```python
from build123d import *

# Parameters (mm, degrees)
SKETCH1_W                                       = 317.5
SKETCH1_H                                       = 50.8
BOSS_EXTRUDE1_DEPTH                             = 6.35
CBORE_FOR_10_SOCKET_HEAD_CAP_SCREW1_D           = 5.1054
CBORE_FOR_10_SOCKET_HEAD_CAP_SCREW1_CBORE_D     = 9.525
CBORE_FOR_10_SOCKET_HEAD_CAP_SCREW1_CBORE_DEPTH = 4.826
CBORE_FOR_10_SOCKET_HEAD_CAP_SCREW2_D           = 5.1054
CBORE_FOR_10_SOCKET_HEAD_CAP_SCREW2_CBORE_D     = 9.525
CBORE_FOR_10_SOCKET_HEAD_CAP_SCREW2_CBORE_DEPTH = 4.826
F_1_4_20_TAPPED_HOLE1_OUTLINE_R                 = 2.5527
F_1_4_20_TAPPED_HOLE1_DEPTH                     = 6.35


# Read off the part's stored shape, not the designer's step: 1/4-20 Tapped Hole1
with BuildPart() as part:
    # Sketch1 → Boss-Extrude1 (new body)
    with BuildSketch(Plane(origin=(0, 0, 0), x_dir=(1, 0, 0), z_dir=(0, 1, 0))):
        Rectangle(SKETCH1_W, SKETCH1_H)
    extrude(amount=BOSS_EXTRUDE1_DEPTH)

    # CBORE for #10 Socket Head Cap Screw1 (through all)
    with Locations(Plane(origin=(0, 6.35, 0), x_dir=(1, 0, 0), z_dir=(0, 1, 0))):
        with Locations((-125.73, -5.08), (19.05, 12.7), (69.85, 12.7), (19.05, -12.7), (69.85, -12.7), (-125.73, 15.24), (-125.73, 5.08), (-125.73, -15.24)):
            CounterBoreHole(CBORE_FOR_10_SOCKET_HEAD_CAP_SCREW1_D / 2, CBORE_FOR_10_SOCKET_HEAD_CAP_SCREW1_CBORE_D / 2, CBORE_FOR_10_SOCKET_HEAD_CAP_SCREW1_CBORE_DEPTH)

    # CBORE for #10 Socket Head Cap Screw2 (through all)
    with Locations(Plane.XZ):
        with Locations((-146.05, 12.7), (-146.05, 0), (-146.05, -12.7), (146.05, 12.7), (146.05, 0), (146.05, -12.7)):
            CounterBoreHole(CBORE_FOR_10_SOCKET_HEAD_CAP_SCREW2_D / 2, CBORE_FOR_10_SOCKET_HEAD_CAP_SCREW2_CBORE_D / 2, CBORE_FOR_10_SOCKET_HEAD_CAP_SCREW2_CBORE_DEPTH)

    # 1/4-20 Tapped Hole1 outline → 1/4-20 Tapped Hole1 (cut)
    with BuildSketch(Plane(origin=(0, 0, 0), x_dir=(1, 0, 0), z_dir=(0, 1, 0))):
        with Locations((-57.15, 20.32)):
            Circle(F_1_4_20_TAPPED_HOLE1_OUTLINE_R)
    extrude(amount=F_1_4_20_TAPPED_HOLE1_DEPTH, mode=Mode.SUBTRACT)


solid = part.part
```
CAD build for the part. Positions are in the model's coordinates, mm. A direction names the side the tool comes from. Round coordinates to 2 decimals unless told otherwise and drop trailing zeros. Write item = value, one per line. Start each with the question number.
Q1. Mould opens along X. For faces 1 (the flat face through (-2, 6.35, 0)), 2 (the cylindrical face through (-148.485, 5.599, 13.467)), 3 (the cylindrical face through (-123.18, 0.75, 4.97)) say: pulls with the +X half, pulls with the -X half, needs draft (parallel to the pull), parting line crosses it, or undercut.
Q2. Drop flat-ended pins along their axis: pin 1 (8.5 mm diameter, centred on x = 19.05, z = 12.7, fed in from +Y); pin 2 (8 mm diameter, centred on x = 146.05, z = -12.7, fed in from -Y). Give the stop position or say it passes through.
Q3. Probe L1, parallel to Z at x = 146.05, y = 1.45; L2, parallel to Z at x = 69.85, y = 4.7; L3, parallel to Z at x = -125.73, y = 2.8. List the from-to ranges inside material, lowest first. Write a range as from..to.
Q4. Which spindle directions (+Z, -Z, +X, -X, +Y, -Y) get a long thin tool onto all of the face, cutting with end or side? Do faces 4 (the flat face through (-123.7, 1.524, 17.3)), 5 (the cylindrical face through (-123.18, 0.75, 15.13)), 6 (the flat face through (-144, 4.826, -15)). Say none if no direction does.
Answers below:
q1.face_1 = needs draft
q1.face_2 = undercut
q1.face_3 = undercut
q2.pin_1 = 1.52
q2.pin_2 = 4.83
q3.L1 = -25.4..-17.46, -7.94..-4.76, 4.76..7.94, 17.46..25.4
q3.L2 = -25.4..-17.46, -7.94..7.94, 17.46..25.4
q3.L3 = -25.4..-20, -10.48..-9.84, -0.32..0.32, 9.84..10.48, 20..25.4
q4.face_4 = +Y
q4.face_5 = +Y, -Y
q4.face_6 = -Y
